For this review, take the finished solid that the model builds, in its own axes (mm). A direction names the side the tool comes from. Coordinates: 2 decimals unless noted, no trailing zeros. Write each loop counter-clockwise with the first axis right and the second up, starting at its lowest first coordinate (ties: lowest second). Pieces come first, ordered by that corner, then holes. Notation, with made-up numbers: (68.5, -2) - (110.5, -2) arc R10 cw to (110.5, 13) - close; hole circle Ø8 at (38, 9.5). An arc over 180 degrees is marked (long way). Use one line per item in the form item = value. Start each with the question number.
1) We need section A-A (z = -5.5). Give the boundary of the cut face in (x, y).
2) Insertion check: P1, Ø1.5, axis at y = 8, z = 1, coming from the -X side; P2, Ø2, axis at x = 6.5, y = 35, coming from the -Z side; P3, Ø5, axis at x = -9, y = 7, coming from the +Z side. Each pin has a flat end and moves straight along its axis. Give the tip position at first contact, or say it passes through.
3) We need section C-C (x = 8.5). Give the boundary of the cut face in (y, z).
4) Mouldability with a two-part tool opening along X and no side actions: class faces 1 (the cylindrical face through (-5.74, 32.47, -4.01)), 2 (the flat face through (-6.501, 32.465, -3.754)), 3 (the flat face through (0, 0, 0)), 4 (the cylindrical face through (-7.735, 32.465, -2.042)) as pulls with the +X half, pulls with the -X half, needs draft (parallel to the pull), parting line crosses it, or undercut.
5) For L1, parallel to Y at x = 8.75, z = 3; L2, parallel to Y at x = 6, z = -9.5; L3, parallel to Y at x = 1.75, z = -0.75, list the stretches that pass through material, from the lowest coordinate up. Write a range as from..to.
6) We need section B-B (x = 0). Give the boundary of the cut face in (y, z), plus the area to 3 significant figures.
7) Tool access review of faces 5 (the flat face through (-3.1, 32.5, -2.6)), 6 (the flat face through (-5, 33, 0)), 7 (the cylindrical face through (9.414, 35.986, 3.374)), 8 (the flat face through (6.489, 32.465, 3.747)), 9 (the cylindrical face through (4.38, 24.93, -8.43)): name each direction out of +Z, -Z, +X, -X, +Y, -Y from which nothing blocks a thin tool from reaching the whole face with its end or side.
8) We need section D-D (y = 11). Give the boundary of the cut face in (x, z).
Autodesk Inventor part; units mm, degrees
ref_plane "YZ Plane" through (0, 0, 0) normal (1, 0, 0) x (0, 1, 0)
ref_plane "XZ Plane" through (0, 0, 0) normal (0, 1, 0) x (-1, 0, 0)
ref_plane "XY Plane" through (0, 0, 0) normal (0, 0, 1) x (1, 0, 0)
sketch "スケッチ1" plane through (0, 0, 0) normal (0, 1, 0) x (-1, 0, 0)
  circle A0 centre (0, 0) radius 12.5
  dimension "d0" = 25
extrude "押し出し1" add sketch "スケッチ1" along normal blind 20
sketch "スケッチ2" plane through (0, 20, 0) normal (0, 1, 0) x (1, 0, 0)
  circle A0 centre (0, 0) radius 9.5
  dimension "d3" = 19
extrude "押し出し2" add sketch "スケッチ2" along normal blind 10
sketch "スケッチ3" plane through (0, 30, 0) normal (0, 1, 0) x (1, 0, 0)
  arc A0 (-6.9282, 4) -> (-8, 0) centre (0, 0) ccw
  line L0 (0, 0) -> (-6.9282, 4) construction
  line L1 (0, 0) -> (-8, 0) construction
  circle A1 centre (0, 0) radius 9.5
  arc A2 (-5.3623, 4.4995) -> (-6.0622, 3.5) centre (0, 0) ccw
  line L2 (0, 0) -> (-5.3623, 4.4995) construction
  line L3 (0, 0) -> (-6.0622, 3.5) construction
  arc A3 (6.9282, -4) -> (8, 0) centre (0, 0) ccw
  line L4 (0, 0) -> (6.9282, -4) construction
  line L5 (0, 0) -> (8, 0) construction
  arc A4 (5.3623, -4.4995) -> (6.0622, -3.5) centre (0, 0) ccw
  line L6 (0, 0) -> (5.3623, -4.4995) construction
  line L7 (0, 0) -> (6.0622, -3.5) construction
  line L8 (-5.3623, 4.4995) -> (0, 0)
  line L9 (-6.9282, 4) -> (0, 0)
  line L10 (-8, 0) -> (0, 0)
  line L11 (0, 0) -> (8, 0)
  line L12 (0, 0) -> (6.9282, -4)
  line L13 (0, 0) -> (5.3623, -4.4995)
  point P0 (-6.0622, 3.5)
  point P1 (6.0622, -3.5)
  dimension "d6" = 8
  dimension "d7" = 30
  dimension "d8" = 7
  dimension "d9" = 10
  dimension "d10" = 8
  dimension "d11" = 30
  dimension "d12" = 7
  dimension "d13" = 10
extrude "押し出し3" add sketch "スケッチ3" along normal blind 5 contours L9 L10 A0 | L11 A3 L12 | L12 A4 L13 | A2 L8 L9
sketch "スケッチ4" plane through (0, 35, 0) normal (0, 1, 0) x (1, 0, 0)
  line L0 (8, 0) -> (0, 0)
  arc A0 (-7.6604, 6.4279) -> (-10, 0) centre (0, 0) ccw
  line L1 (0, 0) -> (-7.6604, 6.4279) construction
  line L2 (0, 0) -> (-10, 0) construction
  line L3 (0, 0) -> (5.3623, -4.4995)
  arc A1 (7.6604, -6.4279) -> (10, 0) centre (0, 0) ccw
  line L4 (0, 0) -> (7.6604, -6.4279) construction
  line L5 (0, 0) -> (10, 0) construction
  line L6 (-7.6604, 6.4279) -> (0, 0)
  line L7 (0, 0) -> (-10, 0)
  line L8 (0, 0) -> (-10, 0)
  line L9 (0, 0) -> (10, 0)
  line L10 (-8, 0) -> (0, 0)
  line L11 (0, 0) -> (7.6604, -6.4279)
  dimension "d16" = 10
  dimension "d17" = 40
  dimension "d18" = 10
  dimension "d19" = 40
extrude "押し出し4" add sketch "スケッチ4" along normal blind 2
sketch "スケッチ5" plane through (0, 37, 0) normal (0, 1, 0) x (1, 0, 0)
  line L0 (0, 0) -> (-8, 0)
  circle A0 centre (0, 0) radius 1
  dimension "d22" = 2
extrude "押し出し5" cut sketch "スケッチ5" against normal blind 7
properties part number "kumi3"
Determined:
q1.outline = (-11.22, 0) - (11.22, 0) - (11.22, 20) - (7.75, 20) - (7.75, 30) - (-7.75, 30) - (-7.75, 20) - (-11.22, 20) - close; (-8.35, 35) - (-6.55, 35) - (-6.55, 37) - (-8.35, 37) - close
q2.P1 = -12.5
q2.P2 = 0
q2.P3 = 10.68
q3.outline = (0, -9.17) - (20, -9.17) - (20, -4.24) - (30, -4.24) - (30, 4.24) - (20, 4.24) - (20, 9.17) - (0, 9.17) - close; (35, 0) - (37, 0) - (37, 5.27) - (35, 5.27) - close
q4.face_1 = undercut
q4.face_2 = undercut
q4.face_3 = needs draft
q4.face_4 = pulls with the -X half
q5.L1 = 0..30, 35..37
q5.L2 = 0..20
q5.L3 = 0..30
q6.outline = (0, -12.5) - (20, -12.5) - (20, -9.5) - (30, -9.5) - (30, 9.5) - (20, 9.5) - (20, 12.5) - (0, 12.5) - close
q6.area = 690 mm²
q7.face_5 = -Z, +X, +Y
q7.face_6 = +Z, -X, +Y
q7.face_7 = +Z, +X, +Y
q7.face_8 = +Z
q7.face_9 = none
q8.outline = circle Ø25 at (0, 0)
